```python
from build123d import *

# Parameters (mm, degrees)
F0_W      = 76.2
F0_H      = 42.164
F1_DEPTH  = 152.4
F3_DEPTH  = 42.165
F5_DEPTH  = 34.29
F7_R      = 11.43
F8_DEPTH  = 4.191
F9_R      = 3.048
F10_DEPTH = 6.35
F12_DEPTH = 6.35
F14_D     = 4.0386


# Not quite as in the source:
# - a pattern or mirror of a feature is missing from the dataset's text; its kind, count and spacing are read off the source's solid


with BuildPart() as f1:
    # F0 (on Top) → F1 (new body)
    with BuildSketch(Plane.XY):
        with Locations((38.1, 21.082)):
            Rectangle(F0_W, F0_H)
    extrude(amount=F1_DEPTH)

    # F2 (on face) → F3 (cut, through all)
    with BuildSketch(Plane.XZ):
        with BuildLine():
            Line((23.1775, 19.431), (76.2, 19.431))
            Line((76.2, 19.431), (76.2, 132.969))
            Line((76.2, 132.969), (23.1775, 132.969))
            ThreePointArc((23.1775, 132.969), (22.0549679849, 132.5040320151), (21.59, 131.3815))
            Line((21.59, 131.3815), (21.59, 21.0185))
            ThreePointArc((21.59, 21.0185), (22.0549679849, 19.8959679849), (23.1775, 19.431))
        make_face()
    extrude(amount=-F3_DEPTH, mode=Mode.SUBTRACT)

    # F4 (on face) → F5 (cut)
    with BuildSketch(Plane.YZ.offset(76.2)):
        with BuildLine():
            Line((36.322, 17.8435), (36.322, 19.431))
            Line((36.322, 19.431), (5.842, 19.431))
            Line((5.842, 19.431), (5.842, 17.8435))
            ThreePointArc((5.842, 17.8435), (6.3069679849, 16.7209679849), (7.4295, 16.256))
            Line((7.4295, 16.256), (10.287, 16.256))
            Line((10.287, 16.256), (10.287, 12.1285))
            ThreePointArc((10.287, 12.1285), (10.7519679849, 11.0059679849), (11.8745, 10.541))
            Line((11.8745, 10.541), (30.2895, 10.541))
            ThreePointArc((30.2895, 10.541), (31.4120320151, 11.0059679849), (31.877, 12.1285))
            Line((31.877, 12.1285), (31.877, 16.256))
            Line((31.877, 16.256), (34.7345, 16.256))
            ThreePointArc((34.7345, 16.256), (35.8570320151, 16.7209679849), (36.322, 17.8435))
        make_face()
    f5 = extrude(amount=-F5_DEPTH, mode=Mode.SUBTRACT)

    # F5_copies: F5 across plane
    add(f5.mirror(Plane.XY.offset(76.2)), mode=Mode.SUBTRACT)

    # F7 (on face) → F8 (cut)
    with BuildSketch(Plane(origin=(0, 0, 0), x_dir=(1, 0, 0), z_dir=(0, 0, -1))):
        with Locations((60.96, -21.082)):
            Circle(F7_R)
    f8 = extrude(amount=-F8_DEPTH, mode=Mode.SUBTRACT)

    # F8_copies: F8 across plane
    add(f8.mirror(Plane.XY.offset(76.2)), mode=Mode.SUBTRACT)

    # F9 (on face) → F10 (cut, through all)
    with BuildSketch(Plane(origin=(0, 0, 4.191), x_dir=(1, 0, 0), z_dir=(0, 0, -1))):
        with Locations((60.96, -21.082)):
            Circle(F9_R)
    f10 = extrude(amount=-F10_DEPTH, mode=Mode.SUBTRACT)

    # F10_copies: F10 across plane
    add(f10.mirror(Plane.XY.offset(76.2)), mode=Mode.SUBTRACT)

    # F11 (on face) → F12 (cut)
    with BuildSketch(Plane(origin=(0, 0, 0), x_dir=(0, -1, 0), z_dir=(-1, 0, 0))):
        with BuildLine():
            Line((-32.639, 6.35), (0, 6.35))
            Line((0, 6.35), (0, 146.05))
            Line((0, 146.05), (-32.639, 146.05))
            ThreePointArc((-32.639, 146.05), (-34.8840640303, 145.1200640303), (-35.814, 142.875))
            Line((-35.814, 142.875), (-35.814, 9.525))
            ThreePointArc((-35.814, 9.525), (-34.8840640303, 7.2799359697), (-32.639, 6.35))
        make_face()
    extrude(amount=-F12_DEPTH, mode=Mode.SUBTRACT)

    # F14 (through all)
    with Locations(Plane(origin=(6.35, 0, 0), x_dir=(0, -1, 0), z_dir=(-1, 0, 0))):
        with Locations((-21.082, 120.65), (-21.082, 31.75)):
            Hole(F14_D / 2)


solid = f1.part
```
Geometry check sheet. Reference: the model listing, model coordinates, mm. A direction names the side the tool comes from. Give positions to 0.01 mm unless a question says otherwise; leave off trailing zeros. Write each loop counter-clockwise with the first axis right and the second up, starting at its lowest first coordinate (ties: lowest second). Pieces come first, ordered by that corner, then holes. Notation, with made-up numbers: (-7, -14) -> (8, -14) arc R11 ccw to (8, -7) -> close; hole circle Ø2 at (26.5, 66.5). An arc over 180 degrees is marked (long way). Use one line per item in the form item = value.
Item 1: Sectioned sample at B-B on z = 89. Enter the section's corners in (x, y).
Results list:
outline = (0, 35.81) -> (6.35, 35.81) -> (6.35, 0) -> (21.59, 0) -> (21.59, 42.16) -> (0, 42.16) -> close
Item 2: Depth check by flat-ended pin: pin 1 Ø5 at (y, z) = (30, 34.5) entering from +X; pin 2 Ø1.2 at (x, z) = (65, 139) entering from -Y; pin 3 Ø3 at (x, z) = (3.5, 51.5) entering from -Y; pin 4 Ø13.5 at (x, y) = (60.96, 21.082) entering from -Z. Enter the tip coordinate at first touch or a pass-through.
Results list:
pin_1 = 21.59
pin_2 = 0
pin_3 = 35.81
pin_4 = 4.19
Item 3: Access from +Z, -Z, +X, -X, +Y, -Y to the whole of each face (thin tool, end or side, straight path). Record for faces 1 (the flat face through (63.3, 23.5, 4.191)), 2 (the flat face through (59, 10.287, 138)), 3 (the flat face through (63.3, 23.5, 148.209)), 4 (the cylindrical face through (3.131, 34.909, 7.305)), 5 (the flat face through (21.59, 21, 77)).
Results list:
face_1 = -Z
face_2 = +X
face_3 = +Z
face_4 = -X, -Y
face_5 = +X, +Y, -Y
Item 4: Mould release check, pull along Z, two halves, no side actions. Record for faces 6 (the cylindrical face through (14.08, 20.64, 118.68)), 7 (the flat face through (38, 21, 0)), 8 (the flat face through (38, 21, 152.4)): released by +Z, released by -Z, zero draft, split by the parting line, or undercut.
Results list:
face_6 = undercut
face_7 = released by -Z
face_8 = released by +Z
Item 5: Scan lines: line 1 (Z direction, x = 46, y = 39.5); line 2 (Z direction, x = 59.5, y = 25.5); line 3 (Y direction, x = 60.96, z = 149.8). Record each from-to range of solid material in increasing order.
Results list:
line_1 = 0 to 19.43, 132.97 to 152.4
line_2 = 4.19 to 10.54, 141.86 to 148.21
line_3 = 0 to 9.65, 32.51 to 42.16
Item 6: Sectioned sample at A-A on z = 120.65. Enter the section's corners in (x, y).
Results list:
outline = (0, 35.81) -> (6.35, 35.81) -> (6.35, 23.1) -> (21.59, 23.1) -> (21.59, 42.16) -> (0, 42.16) -> close; (6.35, 0) -> (21.59, 0) -> (21.59, 19.06) -> (6.35, 19.06) -> close
Item 7: Sectioned sample at C-C on x = 60.96. Count the separate pieces of the cut face and the enclosed holes in it, plus the area to 3 significant figures.
Results list:
separate_pieces = 4
enclosed_holes = 0
area = 934 mm2
